The listing builds one solid part. Answer for the finished solid, in the listing's coordinates (mm). Face numbers are marked on the shaded views. A direction names the side the tool comes from. Give positions to 0.01 mm unless a question says otherwise; leave off trailing zeros. Loops run counter-clockwise (first coordinate to the right, second up) from the corner with the lowest first, then second, coordinate; pieces in that order, holes last. Notation, with made-up numbers: (22, 67) -> (40, 67) arc R37 cw to (40, 105) -> close; hole circle Ø9 at (-34.5, -22.75). An arc over 180 degrees is marked (long way). One line per question, with ' | ' between items. Start each with the question number.
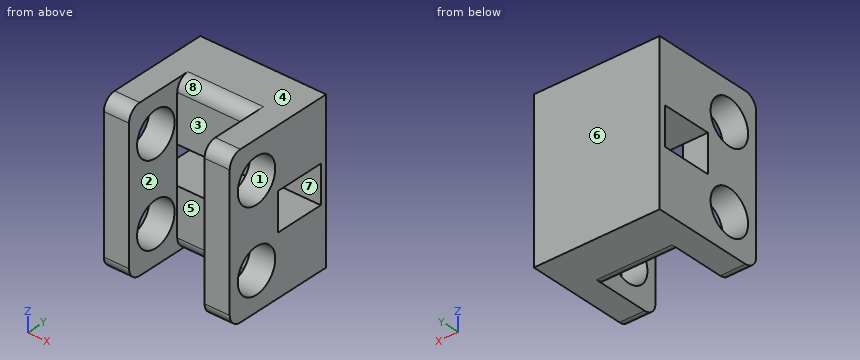
Autodesk Inventor part; units mm, degrees
ref_plane "Work Plane1" through (0, 0, 12.5) normal (0, 0, 1) x (1, 0, 0)
ref_plane "YZ Plane" through (0, 0, 0) normal (1, 0, 0) x (0, 1, 0)
ref_plane "XZ Plane" through (0, 0, 0) normal (0, 1, 0) x (-1, 0, 0)
sketch "Sketch1" plane through (0, 0, 0) normal (0, 0, 1) x (1, 0, 0)
  line L0 (20, 0) -> (20, 18)
  line L1 (20, 18) -> (0, 18)
  line L2 (0, 18) -> (0, 0)
  line L3 (0, 0) -> (4, 0)
  line L4 (4, 0) -> (4, 9)
  line L5 (4, 9) -> (16, 9)
  line L6 (16, 9) -> (16, 0)
  line L7 (16, 0) -> (20, 0)
  point P0 (10, 9)
  point P1 (10, 18)
  dimension "d0" = 18
  dimension "d1" = 20
  dimension "d2" = 9
  dimension "d28" = 12
  dimension "d29" = 4
  dimension "d30" = 4
extrude "Extrusion1" add sketch "Sketch1" along normal blind 25
sketch "Sketch2" plane through (0, 0, 0) normal (-1, 0, 0) x (0, 0, 1)
  line L0 (0, 0) -> (25, 0)
  line L1 (0, 0) -> (0, 18)
  point P0 (6, 5)
  dimension "d10" = 5
  dimension "d11" = 6
hole "Hole1" at (0, 5, 6) direction (1, 0, 0) diameter 7 end through all
ref_plane "Work Plane1" through (0, 0, 12.5) normal (0, 0, 1) x (1, 0, 0)
mirror "Mirror1" about plane through (0, 0, 12.5) normal (0, 0, 1) of "Hole1"
fillet "Fillet1" radius 2 6 edges at (10, 9, 0) (2, 0, 0) (18, 0, 0) (2, 0, 25) (18, 0, 25) (10, 9, 25)
sketch "Sketch3" plane through (20, 18, 25) normal (1, 0, 0) x (0, 0, -1)
  line L0 (9.5, -1) -> (15.5, -1)
  line L1 (15.5, -1) -> (15.5, -9)
  line L2 (15.5, -9) -> (9.5, -9)
  line L3 (9.5, -9) -> (9.5, -1)
  line L4 (25, 0) -> (0, 0)
  line L5 (0, -16) -> (0, 0)
  point P0 (25, -18)
  dimension "d21" = 6
  dimension "d22" = 8
  dimension "d24" = 9
  dimension "d25" = 9.5
extrude "Extrusion2" cut sketch "Sketch3" against normal blind 20
properties part number "Salida"
1. The part is cut by section A-A (z = 19). Write down the section's boundary in (x, y).
2. The part is cut by section C-C (x = 2). Write down the section's boundary in (y, z), plus the area to 3 significant figures.
3. Determine the mould class of the marked faces 1, 2 and 3 for opening direction Y: released by +Y, released by -Y, zero draft, split by the parting line, or undercut.
4. Straight lines are drawn through the part: L1, parallel to Z at x = 1.8, y = 5; L2, parallel to Z at x = 9.5, y = 15.25; L3, parallel to Y at x = 0.95, z = 19. For each, find the intervals that lie inside material, in ascending order.
5. The part is cut by section D-D (y = 5). Write down the section's boundary in (x, z).
6. Each of these flat-tipped pins is pushed along its axis until it touches: pin 1 Ø4 at (x, z) = (13.5, 21) entering from -Y; pin 2 Ø1.8 at (x, z) = (10, 13) entering from -Y; pin 3 Ø5.5 at (y, z) = (5, 6) entering from +X. Where does it stop, or does it pass through?
7. The part is cut by section B-B (y = 14). Write down the section's boundary in (x, z), plus the area to 3 significant figures.
8. For the marked faces 4, 5, 6, 7 and 8, determine the directions among +Z, -Z, +X, -X, +Y, -Y from which every point of the face is accessible in a straight line to the end or side of a thin tool.
Check sheet entries:
1) outline: (0, 0) -> (4, 0) -> (4, 1.5) -> (0, 1.5) -> close; (0, 8.5) -> (4, 8.5) -> (4, 9) -> (16, 9) -> (16, 8.5) -> (20, 8.5) -> (20, 18) -> (0, 18) -> close; (16, 0) -> (20, 0) -> (20, 1.5) -> (16, 1.5) -> close
2) outline: (0, 2) arc R2 ccw to (2, 0) -> (18, 0) -> (18, 25) -> (2, 25) arc R2 ccw to (0, 23) -> close; hole circle Ø7 at (5, 6); hole circle Ø7 at (5, 19); hole (9, 9.5) -> (17, 9.5) -> (17, 15.5) -> (9, 15.5) -> close | area: 323 mm^2
3) face 1: undercut | face 2: zero draft | face 3: released by -Y
4) L1: z = 0 to 2.5, 9.5 to 15.5, 22.5 to 25 | L2: z = 0 to 9.5, 15.5 to 25 | L3: y = 0 to 1.5, 8.5 to 18
5) outline: (0, 0) -> (4, 0) -> (4, 2.5) -> (0, 2.5) -> close; (0, 9.5) -> (4, 9.5) -> (4, 15.5) -> (0, 15.5) -> close; (0, 22.5) -> (4, 22.5) -> (4, 25) -> (0, 25) -> close; (16, 0) -> (20, 0) -> (20, 2.5) -> (16, 2.5) -> close; (16, 9.5) -> (20, 9.5) -> (20, 15.5) -> (16, 15.5) -> close; (16, 22.5) -> (20, 22.5) -> (20, 25) -> (16, 25) -> close
6) pin 1: stops at y = 9 | pin 2: stops at y = 17 | pin 3: passes through
7) outline: (0, 0) -> (20, 0) -> (20, 9.5) -> (0, 9.5) -> close; (0, 15.5) -> (20, 15.5) -> (20, 25) -> (0, 25) -> close | area: 380 mm^2
8) face 4: +Z, +X, -X, +Y, -Y | face 5: +Z, -Z, -Y | face 6: +Z, -Z, +X, -X, +Y | face 7: +X, -X | face 8: +Z, -Y
